For this review, take the finished solid that the model builds, in its own axes (mm). Give positions to 0.01 mm unless a question says otherwise; leave off trailing zeros. Write each loop counter-clockwise with the first axis right and the second up, starting at its lowest first coordinate (ties: lowest second). Pieces come first, ordered by that corner, then holes.
1) We need section B-B on x = 311. Give the boundary of the cut face in (y, z), and give its area (3 significant figures).
2) For P1, Ø8, axis at y = 214, z = 10.5, coming from the -X side, flat-tipped, find the tip position at first contact; note if it passes through.
3) We need section A-A on z = 8.75. Give the number of separate pieces and of enclosed holes in the cut face, and give its area (3 significant figures).
4) Draft analysis for pull direction Y (two halves, no side actions). For faces 1 (the face through (202, 0, 8)), 2 (the face through (379.702, 179.043, 7.888)), 3 (the face through (202, 480, 8)), 4 (the face through (202, 243, 0)), state which applies: pulls with the +Y half, pulls with the -Y half, needs draft (parallel to the pull), parting line crosses it, or undercut.
5) Wall thickness on line 1 along Y through (x, z) = (373, 4); line 2 along Y through (x, z) = (296.5, 4.25); line 3 along X through (y, z) = (54, 7.75): over which ranges is each line inside the solid? List them lowest first.
from build123d import *

# Parameters (mm, degrees)
SKETCH1_W      = 410
SKETCH1_H      = 480
SKETCH1_R      = 15.5
EXTRUDE1_DEPTH = 16


with BuildPart() as part:
    # Sketch1 → Extrude1 (new body)
    with BuildSketch(Plane.XY):
        with Locations((205, 240)):
            Rectangle(SKETCH1_W, SKETCH1_H)
        with Locations((367.4021887, 310.38841599)):
            Circle(SKETCH1_R, mode=Mode.SUBTRACT)
        with Locations((107.261778202, 118.413652083)):
            Circle(SKETCH1_R, mode=Mode.SUBTRACT)
        with Locations((50.874342549, 48.267682131)):
            Circle(SKETCH1_R, mode=Mode.SUBTRACT)
        with Locations(Location((42.5978113, 310.38841599, 0), (0, 0, 180))):
            Circle(SKETCH1_R, mode=Mode.SUBTRACT)
        with Locations(Location((359.125657451, 48.267682131, 0), (0, 0, 180))):
            Circle(SKETCH1_R, mode=Mode.SUBTRACT)
        with Locations(Location((302.738221798, 118.413652083, 0), (0, 0, 180))):
            Circle(SKETCH1_R, mode=Mode.SUBTRACT)
        with Locations(Location((367.4021887, 169.61158401, 0), (0, 0, 180))):
            Circle(SKETCH1_R, mode=Mode.SUBTRACT)
        with Locations(Location((50.874342549, 431.732317869, 0), (0, 0, 180))):
            Circle(SKETCH1_R, mode=Mode.SUBTRACT)
        with Locations(Location((107.261778202, 361.586347917, 0), (0, 0, 180))):
            Circle(SKETCH1_R, mode=Mode.SUBTRACT)
        with Locations((42.5978113, 169.61158401)):
            Circle(SKETCH1_R, mode=Mode.SUBTRACT)
        with Locations((302.738221798, 361.586347917)):
            Circle(SKETCH1_R, mode=Mode.SUBTRACT)
        with Locations((359.125657451, 431.732317869)):
            Circle(SKETCH1_R, mode=Mode.SUBTRACT)
    extrude(amount=EXTRUDE1_DEPTH)


solid = part.part
Results list:
1. outline: (0, 0) - (105.3, 0) - (105.3, 16) - (0, 16) - close; (131.53, 0) - (348.47, 0) - (348.47, 16) - (131.53, 16) - close; (374.7, 0) - (480, 0) - (480, 16) - (374.7, 16) - close
1. area: 6,840 mm2
2. P1: stops at x = 0
3. separate pieces: 1
3. enclosed holes: 12
3. area: 188,000 mm2
4. face 1: pulls with the -Y half
4. face 2: undercut
4. face 3: pulls with the +Y half
4. face 4: needs draft
5. line 1: y = 0 to 41.36, 55.18 to 155.16, 184.07 to 295.93, 324.84 to 424.82, 438.64 to 480
5. line 2: y = 0 to 104.22, 132.6 to 347.4, 375.78 to 480
5. line 3: x = 0 to 36.47, 65.28 to 344.72, 373.53 to 410
